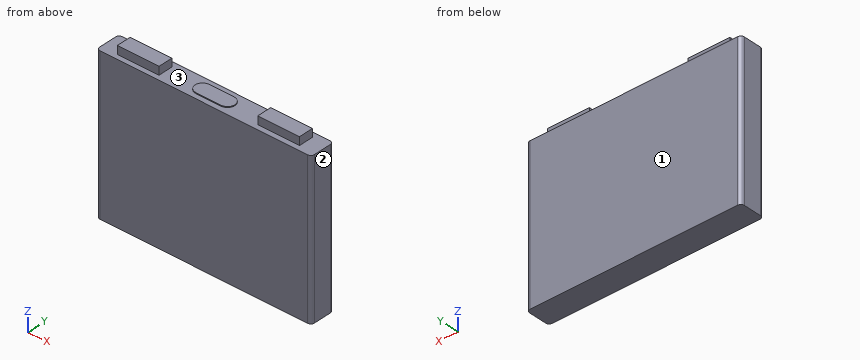
from build123d import *

# Parameters (mm, degrees)
SKETCH1_W           = 120
SKETCH1_H           = 85.5
BOSS_EXTRUDE1_DEPTH = 14
SKETCH2_W           = 23.3
SKETCH2_H           = 8.1
BOSS_EXTRUDE2_DEPTH = 4.5
FILLET2_R           = 2
BOSS_EXTRUDE3_DEPTH = 0.5


with BuildPart() as part:
    # Sketch1 → Boss-Extrude1 (new body)
    with BuildSketch(Plane(origin=(0, 0, 0), x_dir=(1, 0, 0), z_dir=(0, 1, 0))):
        Rectangle(SKETCH1_W, SKETCH1_H)
    extrude(amount=BOSS_EXTRUDE1_DEPTH)

    # Sketch2 → Boss-Extrude2 (add)
    with BuildSketch(Plane.XY.offset(42.75)):
        with Locations((-39.25, 6.894561701)):
            Rectangle(SKETCH2_W, SKETCH2_H)
        with Locations((39.25, 6.894561701)):
            Rectangle(SKETCH2_W, SKETCH2_H)
    extrude(amount=BOSS_EXTRUDE2_DEPTH)

    # Fillet2
    fillet2_edges = [part.edges().sort_by_distance(p)[0] for p in [
        (-60, 14, 0),
        (60, 14, 0),
        (-60, 0, 0),
        (60, 0, 0),
    ]]
    fillet(fillet2_edges, radius=FILLET2_R)

    # Sketch4 → Boss-Extrude3 (add)
    with BuildSketch(Plane.XY.offset(42.75)):
        with BuildLine():
            Line((-7, 2.9), (7, 2.9))
            ThreePointArc((7, 2.9), (11.1, 7), (7, 11.1))
            Line((7, 11.1), (-7, 11.1))
            ThreePointArc((-7, 11.1), (-11.1, 7), (-7, 2.9))
        make_face()
    extrude(amount=BOSS_EXTRUDE3_DEPTH)


solid = part.part
Can you work these out from the model? Positions are in its coordinate system, mm. Face numbers are marked on the shaded views. Coordinates: 2 decimals unless noted, no trailing zeros. Loops run counter-clockwise (first coordinate to the right, second up) from the corner with the lowest first, then second, coordinate; pieces in that order, holes last. Notation, with made-up numbers: (12, 67.25) - (48, 67.25) arc R8 ccw to (48, 73.25) - close; hole circle Ø11 at (77.25, 82). An arc over 180 degrees is marked (long way). Put each result on its own line as item: value. Start each with the question number.
Item 1: If I drill on line 1 along Z through (x, y) = (-18.5, 2.25); line 2 along Z through (x, y) = (2, 6); line 3 along X through (y, z) = (1.25, 28), over which ranges is the centre line in solid material (lowest first)?
Item 2: Suppose I cut it at B-B (y = 7). Please give me the cut outline in (x, z).
Item 3: If we mould it in two halves opening along X, with no side actions, what happens to the marked faces 1, 2 and 3? For each: +X half, -X half, draft (parallel to the pull), parting line (faces both ways), or undercut.
Item 4: For pin 1 (6.5 mm diameter, centred on x = 5.5, y = 7, fed in from +Z); pin 2 (3.5 mm diameter, centred on x = -36.5, z = 45, fed in from -Y); pin 3 (3.5 mm diameter, centred on y = 8, z = 45, fed in from +X), each with a flat end and sliding along its axis, tell me the tip position at first contact or that it passes through.
Item 5: Suppose I cut it at A-A (x = 9.5). Please give me the cut outline in (y, z).
Here are the results:
1. line 1: -42.75 to 42.75
1. line 2: -42.75 to 43.25
1. line 3: -59.85 to 59.85
2. outline: (-60, -42.75) - (60, -42.75) - (60, 42.75) - (50.9, 42.75) - (50.9, 47.25) - (27.6, 47.25) - (27.6, 42.75) - (11.1, 42.75) - (11.1, 43.25) - (-11.1, 43.25) - (-11.1, 42.75) - (-27.6, 42.75) - (-27.6, 47.25) - (-50.9, 47.25) - (-50.9, 42.75) - (-60, 42.75) - close
3. face 1: draft
3. face 2: +X half
3. face 3: undercut
4. pin 1: z = 43.25
4. pin 2: y = 2.84
4. pin 3: x = 50.9
5. outline: (0, -42.75) - (14, -42.75) - (14, 42.75) - (10.25, 42.75) - (10.25, 43.25) - (3.75, 43.25) - (3.75, 42.75) - (0, 42.75) - close
